```python
from build123d import *

# Parameters (mm, degrees)
BOSS_EXTRUDE1_DEPTH = 5
SKETCH7_W           = 14
SKETCH7_H           = 12.5
CUT_EXTRUDE4_DEPTH  = 259.110441478
SKETCH3_W           = 125
SKETCH3_H           = 265
BOSS_EXTRUDE2_DEPTH = 5
SKETCH4_W           = 85
SKETCH4_H           = 40
SKETCH4_H_2         = 139
CUT_EXTRUDE2_DEPTH  = 414.238429965
SKETCH2_R           = 1.5
SKETCH2_W           = 10
SKETCH2_H           = 5
SKETCH2_W_2         = 8
SKETCH2_W_3         = 5
SKETCH2_H_2         = 10
SKETCH2_W_4         = 210
SKETCH2_H_3         = 2
SKETCH2_H_4         = 15
CUT_EXTRUDE1_DEPTH  = 414.238429965
SKETCH5_R           = 1.5
CUT_EXTRUDE3_DEPTH  = 414.238429965
FILLET1_R           = 2
FILLET2_R           = 10
FILLET3_R           = 20
CHAMFER1_SIZE       = 1


with BuildPart() as part:
    # Sketch1 → Boss-Extrude1 (new body)
    with BuildSketch(Plane.XY):
        Polygon((0, 0), (0, 64), (125, 64), (125, 27), (250, 27), (250, 0), align=None)
    extrude(amount=BOSS_EXTRUDE1_DEPTH)

    # Sketch7 → Cut-Extrude4 (cut, through all)
    with BuildSketch(Plane.XY.offset(5)):
        with Locations((54.2, 44.19)):
            Rectangle(SKETCH7_W, SKETCH7_H)
        Polygon((9.74, 28.1), (9.74, 20.4), (34.06, 20.4), (34.06, 28.1), (34.06, 37.6), (9.74, 37.6), align=None)
    extrude(amount=-CUT_EXTRUDE4_DEPTH, mode=Mode.SUBTRACT)

    # Sketch3 → Boss-Extrude2 (add)
    with BuildSketch(Plane.XY.offset(5)):
        with Locations((62.5, 196.5)):
            Rectangle(SKETCH3_W, SKETCH3_H)
    extrude(amount=-BOSS_EXTRUDE2_DEPTH)

    # Sketch4 → Cut-Extrude2 (cut, through all)
    with BuildSketch(Plane.XY.offset(5)):
        with Locations((62.5, 289)):
            Rectangle(SKETCH4_W, SKETCH4_H)
        with Locations((62.5, 154.5)):
            Rectangle(SKETCH4_W, SKETCH4_H_2)
    extrude(amount=-CUT_EXTRUDE2_DEPTH, mode=Mode.SUBTRACT)

    # Sketch2 → Cut-Extrude1 (cut, through all)
    with BuildSketch(Plane.XY.offset(5)):
        with Locations((4.5, 32)):
            Circle(SKETCH2_R)
        with Locations((62.5, 59.5)):
            Circle(SKETCH2_R)
        with Locations(Location((120.5, 32, 0), (0, 0, 180))):
            Circle(SKETCH2_R)
        with Locations((159, 22.5)):
            Circle(SKETCH2_R)
        with Locations(Location((231, 22.5, 0), (0, 0, 180))):
            Circle(SKETCH2_R)
        with Locations((4.5, 109.5)):
            Circle(SKETCH2_R)
        with Locations((4.5, 239.5)):
            Circle(SKETCH2_R)
        with Locations((12, 59.5)):
            Rectangle(SKETCH2_W, SKETCH2_H)
        with Locations((113, 59.5)):
            Rectangle(SKETCH2_W, SKETCH2_H)
        with Locations((241, 22.5)):
            Rectangle(SKETCH2_W_2, SKETCH2_H)
        with Locations((149, 22.5)):
            Rectangle(SKETCH2_W_2, SKETCH2_H)
        with Locations((120.5, 47)):
            Rectangle(SKETCH2_W_3, SKETCH2_H_2)
        with Locations((120.5, 17)):
            Rectangle(SKETCH2_W_3, SKETCH2_H_2)
        with Locations((4.5, 17)):
            Rectangle(SKETCH2_W_3, SKETCH2_H_2)
        with Locations((4.5, 47)):
            Rectangle(SKETCH2_W_3, SKETCH2_H_2)
        with BuildLine():
            Line((173, 22), (217, 22))
            ThreePointArc((217, 22), (225, 30), (217, 38))
            Line((217, 38), (173, 38))
            ThreePointArc((173, 38), (165, 30), (173, 22))
        make_face()
        with Locations((125, 1)):
            Rectangle(SKETCH2_W_4, SKETCH2_H_3)
        with Locations((4.5, 84.5)):
            Rectangle(SKETCH2_W_3, SKETCH2_H_4)
        with Locations((4.5, 264.5)):
            Rectangle(SKETCH2_W_3, SKETCH2_H_4)
        with Locations((4.5, 174.5)):
            Rectangle(SKETCH2_W_3, SKETCH2_H_4)
        with BuildLine():
            Line((61, 82), (64, 82))
            ThreePointArc((64, 82), (65, 81), (64, 80))
            Line((64, 80), (61, 80))
            ThreePointArc((61, 80), (60, 81), (61, 82))
        make_face()
        with BuildLine():
            Line((61, 76), (64, 76))
            ThreePointArc((64, 76), (65, 75), (64, 74))
            Line((64, 74), (61, 74))
            ThreePointArc((61, 74), (60, 75), (61, 76))
        make_face()
    extrude(amount=-CUT_EXTRUDE1_DEPTH, mode=Mode.SUBTRACT)

    # Sketch5 → Cut-Extrude3 (cut, through all)
    with BuildSketch(Plane(origin=(0, 0, 0), x_dir=(-1, 0, 0), z_dir=(0, 0, -1))):
        with Locations((-92.5, 244)):
            Circle(SKETCH5_R)
        with Locations((-62.5, 244)):
            Circle(SKETCH5_R)
        with Locations((-32.5, 244)):
            Circle(SKETCH5_R)
    extrude(amount=-CUT_EXTRUDE3_DEPTH, mode=Mode.SUBTRACT)

    # Fillet1
    fillet1_edges = [part.edges().sort_by_distance(p)[0] for p in [
        (250, 0, 2.5),
        (250, 27, 2.5),
        (0, 0, 2.5),
        (125, 27, 2.5),
        (224.416198487, 27, 2.5),
        (165.583801513, 27, 2.5),
        (230, 0, 2.5),
        (20, 0, 2.5),
    ]]
    fillet(fillet1_edges, radius=FILLET1_R - 0.0001)  # a hair under: the kernel refuses the full size

    # Fillet2
    fillet2_edges = [part.edges().sort_by_distance(p)[0] for p in [
        (20, 269, 2.5),
        (20, 309, 2.5),
        (105, 309, 2.5),
        (105, 269, 2.5),
        (105, 224, 2.5),
        (105, 85, 2.5),
        (20, 85, 2.5),
        (20, 224, 2.5),
    ]]
    fillet(fillet2_edges, radius=FILLET2_R)

    # Fillet3
    fillet3_edges = [part.edges().sort_by_distance(p)[0] for p in [
        (125, 329, 2.5),
        (0, 329, 2.5),
    ]]
    fillet(fillet3_edges, radius=FILLET3_R)

    # Chamfer1
    chamfer1_edges = [part.edges().sort_by_distance(p)[0] for p in [
        (47.2, 37.94, 2.5),
        (61.2, 37.94, 2.5),
    ]]
    chamfer(chamfer1_edges, length=CHAMFER1_SIZE)


solid = part.part
```
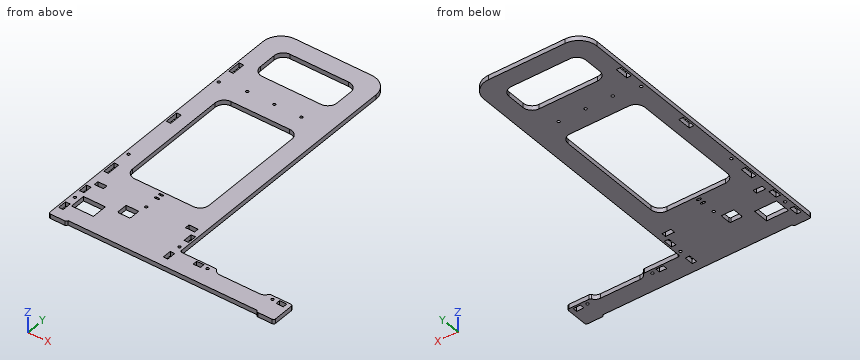
For this review, take the finished solid that the model builds, in its own axes (mm). Coordinates: 2 decimals unless noted, no trailing zeros. Write each loop counter-clockwise with the first axis right and the second up, starting at its lowest first coordinate (ties: lowest second). Pieces come first, ordered by that corner, then holes.
(1) Add section B-B on y = 262.5. Give the boundary of the cut face in (x, z).
(2) Wall thickness on probe 1 along X at (y, z) = (244, 3.75); probe 2 along X at (y, z) = (201.5, 2.15); probe 3 along X at (y, z) = (88, 0.5): over which ranges is each line inside the solid? List them lowest first.
(3) Add section C-C on z = 1.65. Count the separate pieces of the cut face and the enclosed holes in it, then the cut area to 3 significant figures.
(4) For pin 1 Ø2.5 at (x, z) = (4, 2) entering from +Y; pin 2 Ø1.5 at (y, z) = (176, 3.5) entering from +X; pin 3 Ø2.5 at (x, z) = (23.5, 3) entering from -Y, all flat-tipped, find the tip position at first contact; note any pin that passes through.
(5) Add section A-A on y = 187. Give the boundary of the cut face in (x, z), then the cut area to 3 significant figures.
(6) Add section D-D on x = 210. Give the boundary of the cut face in (y, z), then the cut area to 3 significant figures.
Answer sheet:
1. outline: (0, 0) - (2, 0) - (2, 5) - (0, 5) - close; (7, 0) - (125, 0) - (125, 5) - (7, 5) - close
2. probe 1: x = 0 to 31, 34 to 61, 64 to 91, 94 to 125
2. probe 2: x = 0 to 20, 105 to 125
2. probe 3: x = 0 to 2, 7 to 22.86, 102.14 to 125
3. separate pieces: 1
3. enclosed holes: 27
3. area: 27,300 mm2
4. pin 1: stops at y = 322.51
4. pin 2: stops at x = 125
4. pin 3: stops at y = 2
5. outline: (0, 0) - (20, 0) - (20, 5) - (0, 5) - close; (105, 0) - (125, 0) - (125, 5) - (105, 5) - close
5. area: 200 mm2
6. outline: (2, 0) - (22, 0) - (22, 5) - (2, 5) - close
6. area: 100 mm2
